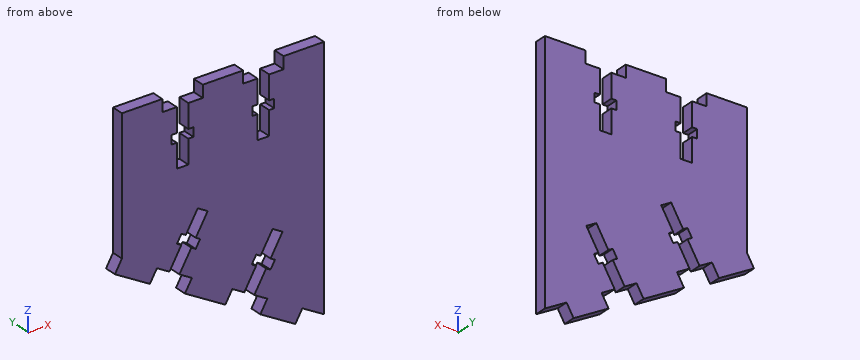
from build123d import *

# Parameters (mm, degrees)
SKETCH1_W           = 50
SKETCH1_H           = 30
SKETCH1_W_2         = 10
SKETCH1_H_2         = 3
BOSS_EXTRUDE1_DEPTH = 3
CUT_EXTRUDE1_DEPTH  = 60.983331018


with BuildPart() as part:
    # Sketch1 → Boss-Extrude1 (new body)
    with BuildSketch(Plane(origin=(0, 0, 0), x_dir=(1, 0, 0), z_dir=(0, 1, 0))):
        Polygon((50, 0), (50, 28.867513459), (0, 0), align=None)
        Polygon((-1.732050808, 3), (0, 0), (8.660254038, 5), (6.92820323, 8), align=None)
        with Locations((25, -15)):
            Rectangle(SKETCH1_W, SKETCH1_H)
        with Locations((5, -31.5)):
            Rectangle(SKETCH1_W_2, SKETCH1_H_2)
        with Locations((25, -31.5)):
            Rectangle(SKETCH1_W_2, SKETCH1_H_2)
        with Locations((45, -31.5)):
            Rectangle(SKETCH1_W_2, SKETCH1_H_2)
        Polygon((15.588457268, 13), (17.320508076, 10), (27.320508076, 15.773502692), (25.588457268, 18.773502692), align=None)
        Polygon((35.980762114, 20.773502692), (44.641016151, 25.773502692), (42.908965344, 28.773502692), (34.248711306, 23.773502692), align=None)
    extrude(amount=BOSS_EXTRUDE1_DEPTH)

    # Sketch2 → Cut-Extrude1 (cut, through all)
    with BuildSketch(Plane(origin=(0, 3, 0), x_dir=(1, 0, 0), z_dir=(0, 1, 0))):
        Polygon((14.224467257, 8.2125), (11.756294856, 6.7875), (14.706294856, 1.677950118), (13.623763102, 1.052950118), (14.723763102, -0.852305771), (15.806294856, -0.227305771), (18.756294856, -5.336855653), (21.224467257, -3.911855653), (18.274467257, 1.197694229), (19.356999012, 1.822694229), (18.256999012, 3.727950118), (17.174467257, 3.102950118), align=None)
        Polygon((32.745265622, 18.905487922), (30.277093221, 17.480487922), (33.211895488, 12.397261285), (32.129363734, 11.772261285), (33.229363734, 9.867005396), (34.311895488, 10.492005396), (37.277093221, 5.356132269), (39.745265622, 6.781132269), (36.780067889, 11.917005396), (37.862599644, 12.542005396), (36.762599644, 14.447261285), (35.680067889, 13.822261285), align=None)
        Polygon((36.425, -16), (33.575, -16), (33.575, -21.9), (32.325, -21.9), (32.325, -24.1), (33.575, -24.1), (33.575, -30), (36.425, -30), (36.425, -24.1), (37.675, -24.1), (37.675, -21.9), (36.425, -21.9), align=None)
        Polygon((16.425, -16), (13.575, -16), (13.575, -21.9), (12.325, -21.9), (12.325, -24.1), (13.575, -24.1), (13.575, -30), (16.425, -30), (16.425, -24.1), (17.675, -24.1), (17.675, -21.9), (16.425, -21.9), align=None)
    extrude(amount=-CUT_EXTRUDE1_DEPTH, mode=Mode.SUBTRACT)


solid = part.part
Input: part model. Units: mm. Frame: model coordinates. Coordinates: 2 decimals unless noted, no trailing zeros. Loops run counter-clockwise (first coordinate to the right, second up) from the corner with the lowest first, then second, coordinate; pieces in that order, holes last. Notation, with made-up numbers: (18.5, 29.5) -> (46.5, 29.5) arc R25 cw to (46.5, 59.5) -> close; hole circle Ø6 at (-39.75, 53.25). An arc over 180 degrees is marked (long way). Write each question's results on one line, items separated by ' | '. Start each with the question number.
Q1. Section C-C, the plane z = -20. Return the cut outline in (x, y), plus the area to 3 significant figures.
Q2. Section B-B, the plane x = 31. Return the cut outline in (y, z).
Q3. Section A-A, the plane z = -9. Return the cut outline in (x, y), plus the area to 3 significant figures.
Q4. Ray query, line 1 (X direction, y = 1.3, z = 26.5) (3 decimals); line 2 (Z direction, x = 37.5, y = 0.45); line 3 (X direction, y = 1.1, z = 15). Return the intervals inside material, ascending. Write a range as from..to.
Q5. Pin query (flat end, axial travel): pin 1 (1.5 mm diameter, centred on x = 18.5, y = 1, fed in from +Z); pin 2 (1.5 mm diameter, centred on y = 1.5, z = -5, fed in from -X); pin 3 (1.5 mm diameter, centred on y = 1.5, z = 31.5, fed in from -X). Return the tip coordinate at first contact, or that it passes through.
Found:
1) outline: (34.64, 0) -> (50, 0) -> (50, 3) -> (34.64, 3) -> close | area: 46.1 mm2
2) outline: (0, -16.23) -> (3, -16.23) -> (3, 30) -> (0, 30) -> close
3) outline: (15.59, 0) -> (35.17, 0) -> (35.17, 3) -> (15.59, 3) -> close; (38.46, 0) -> (50, 0) -> (50, 3) -> (38.46, 3) -> close | area: 93.4 mm2
4) line 1: 0..13.575, 16.425..33.575, 36.425..50 | line 2: -25.65..-13.17, -12.33..-10.67, -5.48..21.9, 24.1..30 | line 3: 0..50
5) pin 1: z = 30 | pin 2: x = 0.43 | pin 3: x = 0
